```python
from build123d import *

# Parameters (mm, degrees)
F0_W     = 31.800013
F0_H     = 15.799999
F1_DEPTH = 9.600006
F2_R     = 2.399995
F3_DEPTH = 1.799999
F4_W     = 29.400012
F4_H     = 13.399999
F4_R     = 3.255
F4_R_2   = 2.399995
F5_DEPTH = 8.600006


with BuildPart() as f1:
    # F0 (on Top) → F1 (new body)
    with BuildSketch(Plane.XY):
        with Locations((15.900006, -7.899999)):
            Rectangle(F0_W, F0_H)
    extrude(amount=-F1_DEPTH)

    # F2 (on Top) → F3 (join)
    with BuildSketch(Plane.XY):
        with Locations((3.999992, -4.000005)):
            Circle(F2_R)
        with Locations((12.000001, -4.000005)):
            Circle(F2_R)
        with Locations((20.000011, -4.000005)):
            Circle(F2_R)
        with Locations((28.00002, -4.000005)):
            Circle(F2_R)
        with Locations((28.00002, -12.000014)):
            Circle(F2_R)
        with Locations((20.000011, -12.000014)):
            Circle(F2_R)
        with Locations((12.000001, -12.000014)):
            Circle(F2_R)
        with Locations((3.999992, -12.000014)):
            Circle(F2_R)
    extrude(amount=F3_DEPTH)

    # F4 (on face) → F5 (cut)
    with BuildSketch(Plane(origin=(0, 0, -9.600006), x_dir=(1, 0, 0), z_dir=(0, 0, -1))):
        with Locations((15.900006, 7.899999)):
            Rectangle(F4_W, F4_H)
        with Locations((7.312597, 8.064775)):
            Circle(F4_R, mode=Mode.SUBTRACT)
        with Locations((15.900006, 8.064775)):
            Circle(F4_R, mode=Mode.SUBTRACT)
        with Locations((24.547525, 8.064775)):
            Circle(F4_R, mode=Mode.SUBTRACT)
        with Locations((7.312597, 8.064775)):
            Circle(F4_R_2)
        with Locations((15.900006, 8.064775)):
            Circle(F4_R_2)
        with Locations((24.547525, 8.064775)):
            Circle(F4_R_2)
    extrude(amount=-F5_DEPTH, mode=Mode.SUBTRACT)


solid = f1.part
```
The listing builds one solid part. Answer for the finished solid, in the listing's coordinates (mm). A direction names the side the tool comes from. Round coordinates to 2 decimals unless told otherwise and drop trailing zeros. Order: outer loops, then holes, each group sorted by start corner. A loop starts at its lowest first (then second) coordinate and runs counter-clockwise, first axis right, second up. Notation, with made-up numbers: (-6, 26.5) -> (51, 26.5) arc R26 cw to (51, 55.5) -> close; hole circle Ø10 at (9, 34). An arc over 180 degrees is marked (long way). Answer as CSV lines item,"result". Start each with the question number.
(1) For a pull along X with two mould halves and no side action, classify faces 1 (the face through (28, -4, 1.8)), 2 (the face through (9.6, -8.79, -5.36)), 3 (the face through (0, -8, -5)) as +X half, -X half, draft (parallel to the pull), parting line (faces both ways), or undercut.
(2) Flat-ended cylindrical pins translate along their axes: pin 1 Ø6 at (x, y) = (15.9, -8.06) entering from +Z; pin 2 Ø3 at (x, y) = (7.31, -8.06) entering from -Z. Find the tip coordinate at first contact, or state that the pin passes through.
(3) A tool of negligible diameter and unlimited length cuts with its end or side. For faces 4 (the face through (25.602, -3.894, 0.887)), 5 (the face through (1.2, -8, -5)), 6 (the face through (4, -4, 1.8)), from which of +Z, -Z, +X, -X, +Y, -Y can it reach the whole face along a straight path? Write none if from no direction.
(4) The part is cut by section D-D (y = -13). Determine the outline of the cut face in (x, z), then the cut area to 3 significant figures.
(5) Find the intervals of material crossed by probe 1 along X at (y, z) = (-1.75, -2.5); probe 2 along Y at (x, z) = (11.5, -3.5); probe 3 along Y at (x, z) = (16, -4.25), in increasing order. Write a range as from..to.
(6) The part is cut by section A-A (z = -4.25). Determine the outline of the cut face in (x, y) (3 decimals), then the cut area to 3 significant figures.
(7) The part is cut by section C-C (z = 0.5). Determine the outline of the cut face in (x, y), then the cut area to 3 significant figures.
(8) The part is cut by section B-B (x = 12). Determine the outline of the cut face in (y, z).
Evaluation:
1,face 1,"draft"
1,face 2,"undercut"
1,face 3,"-X half"
2,pin 1,"z = 0"
2,pin 2,"z = -1"
3,face 4,"+Z"
3,face 5,"-Z"
3,face 6,"+Z, +X, -X, +Y, -Y"
4,outline,"(0, -9.6) -> (1.2, -9.6) -> (1.2, -1) -> (30.6, -1) -> (30.6, -9.6) -> (31.8, -9.6) -> (31.8, 0) -> (30.18, 0) -> (30.18, 1.8) -> (25.82, 1.8) -> (25.82, 0) -> (22.18, 0) -> (22.18, 1.8) -> (17.82, 1.8) -> (17.82, 0) -> (14.18, 0) -> (14.18, 1.8) -> (9.82, 1.8) -> (9.82, 0) -> (6.18, 0) -> (6.18, 1.8) -> (1.82, 1.8) -> (1.82, 0) -> (0, 0) -> close"
4,area,"83.9 mm²"
5,probe 1,"0..1.2, 30.6..31.8"
5,probe 2,"-15.8..-14.6, -1.2..0"
5,probe 3,"-15.8..-14.6, -11.32..-10.46, -5.67..-4.81, -1.2..0"
6,outline,"(0, -15.8) -> (31.8, -15.8) -> (31.8, 0) -> (0, 0) -> close; circle Ø6.51 at (7.313, -8.065); circle Ø6.51 at (15.9, -8.065); circle Ø6.51 at (24.548, -8.065); hole (1.2, -14.6) -> (30.6, -14.6) -> (30.6, -1.2) -> (1.2, -1.2) -> close; hole circle Ø4.8 at (7.313, -8.065); hole circle Ø4.8 at (15.9, -8.065); hole circle Ø4.8 at (24.548, -8.065)"
6,area,"154 mm²"
7,outline,"circle Ø4.8 at (4, -12); circle Ø4.8 at (4, -4); circle Ø4.8 at (12, -12); circle Ø4.8 at (12, -4); circle Ø4.8 at (20, -12); circle Ø4.8 at (20, -4); circle Ø4.8 at (28, -12); circle Ø4.8 at (28, -4)"
7,area,"145 mm²"
8,outline,"(-15.8, -9.6) -> (-14.6, -9.6) -> (-14.6, -1) -> (-1.2, -1) -> (-1.2, -9.6) -> (0, -9.6) -> (0, 0) -> (-1.6, 0) -> (-1.6, 1.8) -> (-6.4, 1.8) -> (-6.4, 0) -> (-9.6, 0) -> (-9.6, 1.8) -> (-14.4, 1.8) -> (-14.4, 0) -> (-15.8, 0) -> close"
